from build123d import *

# Parameters (mm, degrees)
SKETCH1_R           = 10
BOSS_EXTRUDE1_DEPTH = 2
SKETCH2_R           = 5.6
BOSS_EXTRUDE2_DEPTH = 4
SKETCH3_R           = 10
BOSS_EXTRUDE3_DEPTH = 2
CUT_EXTRUDE1_DEPTH  = 17.248076809


with BuildPart() as part:
    # Sketch1 → Boss-Extrude1 (new body)
    with BuildSketch(Plane.XY):
        Circle(SKETCH1_R)
    extrude(amount=BOSS_EXTRUDE1_DEPTH)

    # Sketch2 → Boss-Extrude2 (add)
    with BuildSketch(Plane.XY.offset(2)):
        Circle(SKETCH2_R)
    extrude(amount=BOSS_EXTRUDE2_DEPTH)

    # Sketch3 → Boss-Extrude3 (add)
    with BuildSketch(Plane.XY.offset(6)):
        Circle(SKETCH3_R)
    extrude(amount=BOSS_EXTRUDE3_DEPTH)

    # Sketch6 → Cut-Extrude1 (cut, through all)
    with BuildSketch(Plane.XY.offset(8)):
        with BuildLine():
            Line((1.479493156, 1.56), (-1.479493156, 1.56))
            ThreePointArc((-1.479493156, 1.56), (-0.848996382, -1.975273435), (2.15, 0))
            ThreePointArc((2.15, 0), (1.975273435, 0.848996382), (1.479493156, 1.56))
        make_face()
    extrude(amount=-CUT_EXTRUDE1_DEPTH, mode=Mode.SUBTRACT)


solid = part.part
The listing builds one solid part. Answer for the finished solid, in the listing's coordinates (mm). A direction names the side the tool comes from. Coordinates: 2 decimals unless noted, no trailing zeros. Loops run counter-clockwise (first coordinate to the right, second up) from the corner with the lowest first, then second, coordinate; pieces in that order, holes last. Notation, with made-up numbers: (2.25, 28.25) -> (43.25, 28.25) arc R20 ccw to (43.25, 60.25) -> close; hole circle Ø7 at (32.25, 81). An arc over 180 degrees is marked (long way). Answer in a Markdown table with one row per item. Add a question column.
1. Flat-ended cylindrical pins translate along their axes: P1, Ø2.5, axis at x = 0, y = 0, coming from the +Z side; P2, Ø1.5, axis at x = 0.5, z = 4.5, coming from the -Y side; P3, Ø3, axis at y = 7.5, z = 1.5, coming from the -X side; P4, Ø1, axis at y = 0, z = 4.5, coming from the -X side. Find the tip coordinate at first contact, or state that the pin passes through.
2. The part is cut by section B-B, the plane y = -6.75. Write down the section's boundary in (x, z), then the cut area to 3 significant figures.
3. Consider line 1 (Z direction, x = 3.5, y = 6.5); line 2 (Y direction, x = 0, z = 3.75); line 3 (Y direction, x = 1.25, z = 4.25). Determine where each line is inside the solid, lowest interval first. Write a range as [from, to].
4. Determine the mould class of faces 3 (the flat face through (0, 2, 8)), 4 (the cylindrical face through (-5.595, 0.246, 3.972)), 5 (the flat face through (0, 1.56, 4)) for opening direction Z: +Z half, -Z half, draft (parallel to the pull), parting line (faces both ways), or undercut.
5. The part is cut by section D-D, the plane z = 5. Write down the section's boundary in (x, y).
6. The part is cut by section C-C, the plane x = 0. Write down the section's boundary in (y, z), then the cut area to 3 significant figures.
7. The part is cut by section A-A, the plane x = -6.25. Write down the section's boundary in (y, z).
8. For faces 1 (the cylindrical face through (-2.17, -9.76, 0.99)), 2 (the flat face through (4.3, -4.3, 2)), determine the directions among +Z, -Z, +X, -X, +Y, -Y from which every point of the face is accessible in a straight line to the end or side of a thin tool.
Answer below:
| question | item | result |
|---|---|---|
| 1 | P1 | through |
| 1 | P2 | y = -5.6 |
| 1 | P3 | x = -8 |
| 1 | P4 | x = -5.6 |
| 2 | outline | (-7.38, 0) -> (7.38, 0) -> (7.38, 2) -> (-7.38, 2) -> close; (-7.38, 6) -> (7.38, 6) -> (7.38, 8) -> (-7.38, 8) -> close |
| 2 | area | 59.0 mm2 |
| 3 | line 1 | [0, 2], [6, 8] |
| 3 | line 2 | [-5.6, -2.15], [1.56, 5.6] |
| 3 | line 3 | [-5.46, -1.75], [1.56, 5.46] |
| 4 | face 3 | +Z half |
| 4 | face 4 | undercut |
| 4 | face 5 | draft |
| 5 | outline | circle Ø11.2 at (0, 0); hole (-1.48, 1.56) arc R2.15 ccw (long way) to (1.48, 1.56) -> close |
| 6 | outline | (-10, 0) -> (-2.15, 0) -> (-2.15, 8) -> (-10, 8) -> (-10, 6) -> (-5.6, 6) -> (-5.6, 2) -> (-10, 2) -> close; (1.56, 0) -> (10, 0) -> (10, 2) -> (5.6, 2) -> (5.6, 6) -> (10, 6) -> (10, 8) -> (1.56, 8) -> close |
| 6 | area | 95.1 mm2 |
| 7 | outline | (-7.81, 0) -> (7.81, 0) -> (7.81, 2) -> (-7.81, 2) -> close; (-7.81, 6) -> (7.81, 6) -> (7.81, 8) -> (-7.81, 8) -> close |
| 8 | face 1 | +Z, -Z |
| 8 | face 2 | none |
